The listing builds one solid part. Answer for the finished solid, in the listing's coordinates (mm). Give positions to 0.01 mm unless a question says otherwise; leave off trailing zeros. Order: outer loops, then holes, each group sorted by start corner. A loop starts at its lowest first (then second) coordinate and runs counter-clockwise, first axis right, second up. Notation, with made-up numbers: M 41,74 L 54,74 A26 ccw 54,93 Z; hole C 51.5,89 d4. An arc over 180 degrees is marked long. Answer as a JSON object with one key per item and string values. Group by question number.
```python
from build123d import *

# Parameters (mm, degrees)
ESQUISSE2_R             = 130
BOSS_EXTRU_1_DEPTH      = 15
ESQUISSE3_R             = 35
ENL_V_MAT_EXTRU_1_DEPTH = 15
ESQUISSE4_R             = 3
ENL_V_MAT_EXTRU_3_DEPTH = 24


with BuildPart() as part:
    # Esquisse2 → Boss.-Extru.1 (new body)
    with BuildSketch(Plane(origin=(0, 0, 0), x_dir=(0, 0, -1), z_dir=(1, 0, 0))):
        Circle(ESQUISSE2_R)
    extrude(amount=BOSS_EXTRU_1_DEPTH)

    # Esquisse3 → Enlèv. mat.-Extru.1 (cut)
    with BuildSketch(Plane(origin=(15, 0, 0), x_dir=(0, 0, -1), z_dir=(1, 0, 0))):
        with Locations((0, 85)):
            Circle(ESQUISSE3_R)
        with Locations((85, 0)):
            Circle(ESQUISSE3_R)
        with Locations((0, -85)):
            Circle(ESQUISSE3_R)
        with Locations((-85, 0)):
            Circle(ESQUISSE3_R)
    extrude(amount=-ENL_V_MAT_EXTRU_1_DEPTH, mode=Mode.SUBTRACT)

    # Esquisse4 → Enlèv. mat.-Extru.3 (cut)
    with BuildSketch(Plane(origin=(15, 0, 0), x_dir=(0, 0, -1), z_dir=(1, 0, 0))):
        Circle(ESQUISSE4_R)
    extrude(amount=-ENL_V_MAT_EXTRU_3_DEPTH, mode=Mode.SUBTRACT)


solid = part.part
```
Item 1: Consider probe 1 along Y at (x, z) = (11.25, 0); probe 2 along Z at (x, y) = (13.75, 25); probe 3 along Z at (x, y) = (4.5, -25.5). Determine where each line is inside the solid, lowest interval first. Write a range as from..to.
Item 2: Section A-A (z = 0) is taken. Determine the outline of the cut face in (x, y).
Item 3: Section C-C (x = 10.75) is taken. Determine the outline of the cut face in (y, z), and give its area (3 significant figures).
Item 4: Section D-D (z = 85) is taken. Determine the outline of the cut face in (x, y).
Item 5: Determine the mould class of faces 1 (the cylindrical face through (8, 0, 3)), 2 (the flat face through (15, 2, -27)), 3 (the cylindrical face through (7.395, 39.048, -123.997)) for opening direction Y: released by +Y, released by -Y, zero draft, split by the parting line, or undercut.
Item 6: Flat-ended cylindrical pins translate along their axes: P1, Ø2, axis at x = 5.5, z = -91, coming from the -Y side; P2, Ø5, axis at y = 0, z = 0, coming from the -X side; P3, Ø3, axis at x = 7.5, z = -26, coming from the +Y side; P4, Ø8, axis at x = 12, y = 8, coming from the -Z side. Find the tip coordinate at first contact, or state that the pin passes through.
Values found:
{
 "1": {"probe 1": "y = -130..-120, -50..-3, 3..50, 120..130", "probe 2": "z = -127.57..-109.49, -60.51..60.51, 109.49..127.57", "probe 3": "z = -127.47..-108.97, -61.03..61.03, 108.97..127.47"},
 "2": {"outline": "M 0,-130 L 15,-130 L 15,-120 L 0,-120 Z; M 0,-50 L 15,-50 L 15,-3 L 0,-3 Z; M 0,3 L 15,3 L 15,50 L 0,50 Z; M 0,120 L 15,120 L 15,130 L 0,130 Z"},
 "3": {"outline": "C 0,0 d260; hole C -85,0 d70; hole C 0,-85 d70; hole C 0,85 d70; hole C 0,0 d6; hole C 85,0 d70", "area": "37,700 mm^2"},
 "4": {"outline": "M 0,-98.36 L 15,-98.36 L 15,-35 L 0,-35 Z; M 0,35 L 15,35 L 15,98.36 L 0,98.36 Z"},
 "5": {"face 1": "undercut", "face 2": "zero draft", "face 3": "split by the parting line"},
 "6": {"P1": "stops at y = -93.81", "P2": "passes through", "P3": "stops at y = 127.67", "P4": "stops at z = -129.94"}
}
